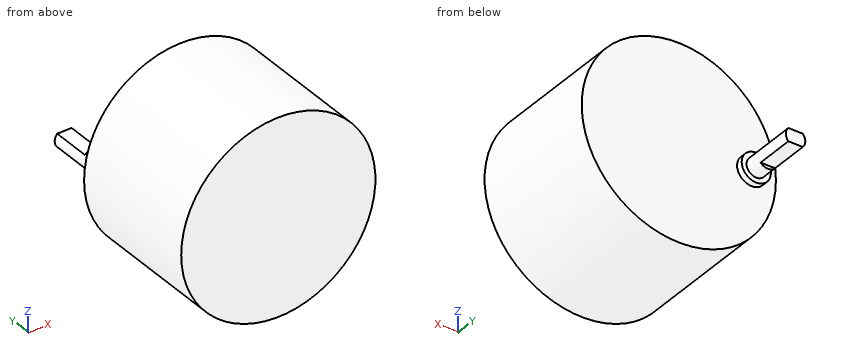
Autodesk Inventor part; units mm, degrees
ref_plane "YZ Plane" through (0, 0, 0) normal (1, 0, 0) x (0, 1, 0)
ref_plane "XZ Plane" through (0, 0, 0) normal (0, 1, 0) x (-1, 0, 0)
ref_plane "XY Plane" through (0, 0, 0) normal (0, 0, 1) x (1, 0, 0)
sketch "Sketch1" plane through (0, 0, 0) normal (0, 1, 0) x (-1, 0, 0)
  circle A0 centre (0, 0) radius 15
  line L0 (-7.5, 13) -> (-7.4833, 13)
  line L1 (7.4833, 13) -> (7.5, 13)
  point P0 (0, 15)
  dimension "d0" = 30
extrude "Extrusion1" add sketch "Sketch1" along normal blind 21
sketch "Sketch2" plane through (0, 21, 0) normal (0, 1, 0) x (1, 0, 0)
  circle A0 centre (-11.25, 0) radius 2.25
  circle A1 centre (0, 0) radius 15
  dimension "d3" = 4.5
  dimension "d4" = 1.5
extrude "Extrusion2" add sketch "Sketch2" along normal blind 1 contours A0
sketch "Sketch3" plane through (-11.25, 22, 0) normal (0, 1, 0) x (1, 0, 0)
  circle A0 centre (0, 0) radius 1.5
  point P0 (11.25, 0)
  dimension "d7" = 3
extrude "Extrusion3" add sketch "Sketch3" along normal blind 2.5
sketch "Sketch4" plane through (-11.25, 24.5, 0) normal (0, 1, 0) x (1, 0, 0)
  line L0 (1.118, -1) -> (-1.118, -1)
  line L1 (-1.118, 1) -> (1.118, 1)
  line L2 (1.5, -1) -> (-1.882, 1) construction
  line L3 (-1.882, -1) -> (1.0655, 1.0558) construction
  circle A0 centre (0, 0) radius 1.5
  point P0 (11.25, 0)
  point P1 (-0.3302, 0.0823)
  dimension "d10" = 3
  dimension "d11" = 0.5
  dimension "d12" = 0.5
extrude "Extrusion4" add sketch "Sketch4" along normal blind 6 contours L0 A0 L1
properties part number "stepperMotor"
Part model, mm, in its own coordinate system. Give positions to 0.01 mm unless a question says otherwise; leave off trailing zeros. Write each loop counter-clockwise with the first axis right and the second up, starting at its lowest first coordinate (ties: lowest second). Pieces come first, ordered by that corner, then holes.
1) Cut at C-C on y = 25. Write the cut outline in (x, z), then the cut area to 3 significant figures.
Resolved:
outline: (-12.37, -1) - (-10.13, -1) arc R1.5 ccw to (-10.13, 1) - (-12.37, 1) arc R1.5 ccw to start
area: 5.52 mm2
2) Probe L1, parallel to Y at x = 6.5, z = -3.75; L2, parallel to Z at x = 0, y = 7; L3, parallel to X at y = 10, z = -6.5. List the from-to ranges inside material, lowest first.
Resolved:
L1: y = 0 to 21
L2: z = -15 to 15
L3: x = -13.52 to 13.52
3) Cut at B-B on x = -11.25. Write the cut outline in (y, z).
Resolved:
outline: (0, -9.92) - (21, -9.92) - (21, -2.25) - (22, -2.25) - (22, -1.5) - (24.5, -1.5) - (24.5, -1) - (30.5, -1) - (30.5, 1) - (24.5, 1) - (24.5, 1.5) - (22, 1.5) - (22, 2.25) - (21, 2.25) - (21, 9.92) - (0, 9.92) - close
4) Cut at A-A on z = 0. Write the cut outline in (x, y), then the cut area to 3 significant figures.
Resolved:
outline: (-15, 0) - (15, 0) - (15, 21) - (-9, 21) - (-9, 22) - (-9.75, 22) - (-9.75, 30.5) - (-12.75, 30.5) - (-12.75, 22) - (-13.5, 22) - (-13.5, 21) - (-15, 21) - close
area: 660 mm2
5) Pin check, flat tips, straight feed: pin 1 (15 mm diameter, centred on x = 1, z = -1.5, fed in from +Y); pin 2 (8 mm diameter, centred on x = 6, y = 20.5, fed in from -Z); pin 3 (2.5 mm diameter, centred on x = -11, y = 26.5, fed in from -Z). Stop position of each tip, or through.
Resolved:
pin 1: stops at y = 21
pin 2: stops at z = -14.87
pin 3: stops at z = -1
6) Cut at D-D on z = -12. Write the cut outline in (x, y).
Resolved:
outline: (-9, 0) - (9, 0) - (9, 21) - (-9, 21) - close
